Model file for the job. Use its own axes, mm. A direction names the side the tool comes from. Give positions to 0.01 mm unless a question says otherwise; leave off trailing zeros. Write each loop counter-clockwise with the first axis right and the second up, starting at its lowest first coordinate (ties: lowest second). Pieces come first, ordered by that corner, then holes. Notation, with made-up numbers: (63.25, -27) - (111.25, -27) arc R22 ccw to (111.25, -5) - close; hole circle Ø11 at (87.5, 3). An arc over 180 degrees is marked (long way). Use CSV: the item, a comma, the result in double quotes.
from build123d import *

# Parameters (mm, degrees)
EXTRUDE006_DEPTH                     = 2
EXTRUDE006_ONTO_SKETCH006_ROLL_ANGLE = 90
EXTRUDE006_PLACEMENT_ANGLE           = 90
SKETCH_W                             = 14.047477
SKETCH_H                             = 45.6
EXTRUDE004_DEPTH                     = 10
SKETCH002_R                          = 1.2
EXTRUDE001_DEPTH                     = 2
EXTRUDE005_DEPTH                     = 10
EXTRUDE003_DEPTH                     = 0.7
EXTRUDE003_DEPTH_BACK                = 0.2
FILLET_R                             = 0.2
CHAMFER_SIZE                         = 0.2
EXTRUDE002_DEPTH                     = 2
EXTRUDE_DEPTH                        = 1.6
EXTRUDE_DEPTH_BACK                   = 6.8


with BuildPart() as extrude006:
    # Sketch006 as drawn → Extrude006 (new, symmetric)
    with BuildSketch(Plane.XY):
        Polygon((-3.8, 0), (-2.9, 0.8), (2.9, 0.8), (3.8, 0), align=None)
    extrude(amount=EXTRUDE006_DEPTH, both=True)


with BuildPart() as extrude006_1:
    # Extrude006 onto Sketch006 roll: moved
    add(extrude006.part.rotate(Axis((0, 0, 0), (1, 0, 0)), EXTRUDE006_ONTO_SKETCH006_ROLL_ANGLE))


with BuildPart() as extrude006_2:
    # Extrude006 onto Sketch006 placement: moved
    add(extrude006_1.part)


with BuildPart() as extrude006_3:
    # Extrude006 placement: moved
    add(extrude006_2.part.moved(Location((50, 9.5, -6.8))).rotate(Axis((50, 9.5, -6.8), (0, 0, 1)), EXTRUDE006_PLACEMENT_ANGLE))


with BuildPart() as extrude004:
    # Sketch → Extrude004 (new body)
    with BuildSketch(Plane.XY):
        with Locations((51.252235, 25)):
            Rectangle(SKETCH_W, SKETCH_H)
    extrude(amount=EXTRUDE004_DEPTH)


with BuildPart() as extrude001:
    # Sketch002 → Extrude001 (new body)
    with BuildSketch(Plane.XY):
        with BuildLine():
            Line((4.8, 47), (4.8, 51))
            Line((4.8, 51), (9.2, 51))
            Line((9.2, 51), (9.2, 47.000001))
            ThreePointArc((4.8, 47), (7, 44.8), (9.2, 47.000001))
        make_face()
        with Locations((7, 47)):
            Circle(SKETCH002_R, mode=Mode.SUBTRACT)
        with BuildLine():
            ThreePointArc((9.2, 3), (7, 5.2), (4.8, 3))
            Line((4.8, 3), (4.8, -1))
            Line((4.8, -1), (9.2, -1))
            Line((9.2, -1), (9.2, 3))
        make_face()
        with Locations((7, 3)):
            Circle(SKETCH002_R, mode=Mode.SUBTRACT)
        with BuildLine():
            Line((40.8, 47), (40.8, 51))
            Line((40.8, 51), (45.2, 51))
            Line((45.2, 51), (45.2, 46.999987))
            ThreePointArc((40.8, 47), (42.999993, 44.8), (45.2, 46.999987))
        make_face()
        with Locations((43, 47)):
            Circle(SKETCH002_R, mode=Mode.SUBTRACT)
        with BuildLine():
            ThreePointArc((45.2, 3), (43, 5.2), (40.8, 3))
            Line((40.8, 3), (40.8, -1))
            Line((40.8, -1), (45.2, -1))
            Line((45.2, -1), (45.2, 3))
        make_face()
        with Locations((43, 3)):
            Circle(SKETCH002_R, mode=Mode.SUBTRACT)
    extrude(amount=-EXTRUDE001_DEPTH)


with BuildPart() as extrude005:
    # Sketch005 → Extrude005 (new body)
    with BuildSketch(Plane.XY):
        Polygon((8, 53), (8, 45), (-3, 45), (-3, 5), (8, 5), (8, -3), (42, -3), (42, 5), (53, 5), (53, 45), (42, 45), (42, 53), align=None)
    extrude(amount=EXTRUDE005_DEPTH)


with BuildPart() as cut003:
    # Sketch004 → Extrude003 (new body, two sides)
    with BuildSketch(Plane.XY) as extrude003_sk:
        with BuildLine():
            Line((2.3, 50.6), (47.7, 50.6))
            ThreePointArc((50.6, 47.7), (49.75061, 49.75061), (47.7, 50.6))
            Line((50.6, 47.7), (50.6, 2.3))
            ThreePointArc((47.7, -0.6), (49.75061, 0.24939), (50.6, 2.3))
            Line((47.7, -0.6), (2.3, -0.6))
            ThreePointArc((-0.6, 2.3), (0.24939, 0.24939), (2.3, -0.6))
            Line((-0.6, 2.3), (-0.6, 47.7))
            ThreePointArc((2.3, 50.6), (0.24939, 49.75061), (-0.6, 47.7))
        make_face()
        with BuildLine():
            Line((2.3, 50), (47.7, 50))
            ThreePointArc((50, 47.7), (49.326346, 49.326346), (47.7, 50))
            Line((50, 47.7), (50, 2.3))
            ThreePointArc((47.7, 0), (49.326346, 0.673654), (50, 2.3))
            Line((47.7, 0), (2.3, 0))
            ThreePointArc((0, 2.3), (0.673654, 0.673654), (2.3, 0))
            Line((0, 2.3), (0, 47.7))
            ThreePointArc((2.3, 50), (0.673654, 49.326346), (0, 47.7))
        make_face(mode=Mode.SUBTRACT)
    extrude(amount=EXTRUDE003_DEPTH)
    extrude(extrude003_sk.sketch, amount=-EXTRUDE003_DEPTH_BACK)


with BuildPart() as cut003_1:
    # Extrude003 placement: moved
    add(cut003.part.moved(Location((0, 0, 1.6))))

    # Fillet
    fillet_edges = [cut003_1.edges().sort_by_distance(p)[0] for p in [
        (-0.6, 25, 2.3),
        (0.24939, 49.75061, 2.3),
        (25, 50.6, 2.3),
        (49.75061, 49.75061, 2.3),
        (50.6, 25, 2.3),
        (49.75061, 0.24939, 2.3),
        (25, -0.6, 2.3),
        (0.24939, 0.24939, 2.3),
    ]]
    fillet(fillet_edges, radius=FILLET_R)

    # Chamfer
    chamfer_edges = [cut003_1.edges().sort_by_distance(p)[0] for p in [
        (0, 25, 1.4),
        (0.673654, 49.326346, 1.4),
        (25, 50, 1.4),
        (49.326346, 49.326346, 1.4),
        (50, 25, 1.4),
        (49.326346, 0.673654, 1.4),
        (25, 0, 1.4),
        (0.673654, 0.673654, 1.4),
    ]]
    chamfer(chamfer_edges, length=CHAMFER_SIZE)

    # Cut003: cut Extrude005
    add(extrude005.part, mode=Mode.SUBTRACT)


with BuildPart() as extrude002:
    # Sketch003 → Extrude002 (new body)
    with BuildSketch(Plane.XY):
        with BuildLine():
            Line((2.3, 51.1), (9, 51.1))
            Line((9, 44), (9, 51.1))
            Line((-1.1, 44), (9, 44))
            Line((-1.1, 44), (-1.1, 47.654452))
            ThreePointArc((2.3, 51.1), (-0.12032, 50.088024), (-1.1, 47.654452))
        make_face()
        with BuildLine():
            Line((51.1, 47.699699), (51.1, 44))
            Line((41, 44), (51.1, 44))
            Line((41, 51.1), (41, 44))
            Line((41, 51.1), (47.698586, 51.1))
            ThreePointArc((51.1, 47.699699), (50.103681, 50.104468), (47.698586, 51.1))
        make_face()
        with BuildLine():
            Line((47.6997, -1.1), (41, -1.1))
            Line((41, -1.1), (41, 6))
            Line((41, 6), (51.1, 6))
            Line((51.1, 6), (51.1, 2.297304))
            ThreePointArc((47.6997, -1.1), (50.103016, -0.105134), (51.1, 2.297304))
        make_face()
        with BuildLine():
            Line((-1.1, 2.300296), (-1.1, 6))
            Line((-1.1, 6), (9, 6))
            Line((9, 6), (9, -1.1))
            Line((9, -1.1), (2.294563, -1.1))
            ThreePointArc((-1.1, 2.300296), (-0.106103, -0.10205), (2.294563, -1.1))
        make_face()
    extrude(amount=-EXTRUDE002_DEPTH)


with BuildPart() as extrude002_1:
    # Extrude002 placement: moved
    add(extrude002.part.moved(Location((0, 0, -5.6))))


with BuildPart() as cut004:
    # Sketch001 → Extrude (new body, two sides)
    with BuildSketch(Plane.XY) as extrude_sk:
        with BuildLine():
            Line((2.3, 52), (47.7, 52))
            ThreePointArc((52, 47.7), (50.740559, 50.740559), (47.7, 52))
            Line((52, 47.7), (52, 2.3))
            ThreePointArc((47.7, -2), (50.740559, -0.740559), (52, 2.3))
            Line((47.7, -2), (2.3, -2))
            ThreePointArc((-2, 2.3), (-0.740559, -0.740559), (2.3, -2))
            Line((-2, 2.3), (-2, 47.7))
            ThreePointArc((2.3, 52), (-0.740559, 50.740559), (-2, 47.7))
        make_face()
        with BuildLine():
            Line((2.3, 50.1), (47.7, 50.1))
            ThreePointArc((50.1, 47.7), (49.397056, 49.397056), (47.7, 50.1))
            Line((50.1, 47.7), (50.1, 2.3))
            ThreePointArc((47.7, -0.1), (49.397056, 0.602944), (50.1, 2.3))
            Line((47.7, -0.1), (2.3, -0.1))
            ThreePointArc((-0.1, 2.3), (0.602944, 0.602944), (2.3, -0.1))
            Line((-0.1, 2.3), (-0.1, 47.7))
            ThreePointArc((2.3, 50.1), (0.602944, 49.397056), (-0.1, 47.7))
        make_face(mode=Mode.SUBTRACT)
    extrude(amount=EXTRUDE_DEPTH)
    extrude(extrude_sk.sketch, amount=-EXTRUDE_DEPTH_BACK)

    # Cut002: cut Extrude002
    add(extrude002_1.part, mode=Mode.SUBTRACT)

    # Fusion001: union Cut003
    add(cut003_1.part)

    # Fusion002: union Extrude001
    add(extrude001.part)

    # Cut: cut Extrude004
    add(extrude004.part, mode=Mode.SUBTRACT)

    # Cut004: cut Extrude006
    add(extrude006_3.part, mode=Mode.SUBTRACT)


solid = cut004.part
(1) 3-axis set-ups, long thin cutter, end or side, ignore diameter. For faces 1 (the face through (50.71, -0.77, -2.54)), 2 (the face through (50.1, 25, -3)), 3 (the face through (49, 50, -5.6)): which of +Z, -Z, +X, -X, +Y, -Y reach the whole face in a straight line?
Checked values:
face 1,"+Z, -Z, +X, -Y"
face 2,"+Z, -Z"
face 3,"-Z"
(2) Saw through at D-D, the plane x = 38.5. List the corners of the cut face in (y, z).
Checked values:
outline,"(-2, -6.8) - (-0.1, -6.8) - (-0.1, 1.6) - (-2, 1.6) - close; (50.1, -6.8) - (52, -6.8) - (52, 1.6) - (50.1, 1.6) - close"
(3) Saw through at A-A, the plane y = 9.5. List the corners of the cut face in (x, z), then the cut area to 3 significant figures.
Checked values:
outline,"(-2, -6.8) - (-0.1, -6.8) - (-0.1, 1.6) - (-2, 1.6) - close; (50.1, -6) - (52, -6) - (52, 0) - (50.1, 0) - close"
area,"27.4 mm^2"
(4) Saw through at B-B, the plane x = 46. List the corners of the cut face in (y, z), then the cut area to 3 significant figures.
Checked values:
outline,"(-2, -6.8) - (-1.1, -6.8) - (-1.1, -5.6) - (-0.1, -5.6) - (-0.1, 1.5) - (0, 1.6) - (0, 2.3) - (-0.4, 2.3) arc R0.2 ccw to (-0.6, 2.1) - (-0.6, 1.6) - (-2, 1.6) - close; (50, 1.6) - (50.1, 1.5) - (50.1, -5.6) - (51.1, -5.6) - (51.1, -6.8) - (52, -6.8) - (52, 1.6) - (50.6, 1.6) - (50.6, 2.1) arc R0.2 ccw to (50.4, 2.3) - (50, 2.3) - close"
area,"30.4 mm^2"
(5) Flat gauge pins, fed straight in: P1, Ø0.6, axis at x = 51.5, z = 1.5, coming from the -Y side; P2, Ø2, axis at x = 7.5, y = 4, coming from the -Z side; P3, Ø0.5, axis at y = -0.5, z = 2, coming from the +X side; P4, Ø1.9, axis at x = 7, y = 3, coming from the -Z side. Where does each tip first touch, or does it go through?
Checked values:
P1,"stops at y = -0.2"
P2,"stops at z = -2"
P3,"stops at x = 49.08"
P4,"passes through"
(6) Pull direction X, two halves, no side cores. Call faces 4 (the face through (-1.1, 4, -6)), 5 (the face through (49.7, 0.2, 1.9)), 6 (the face through (51, 9, -6)): released by +X, released by -X, zero draft, split by the parting line, or undercut.
Checked values:
face 4,"undercut"
face 5,"released by +X"
face 6,"zero draft"
(7) Saw through at C-C, the plane z = -4.75. List the corners of the cut face in (x, y).
Checked values:
outline,"(-2, 2.3) arc R4.3 ccw to (2.3, -2) - (47.7, -2) arc R4.3 ccw to (52, 2.3) - (52, 47.7) arc R4.3 ccw to (47.7, 52) - (2.3, 52) arc R4.3 ccw to (-2, 47.7) - close; hole (-0.1, 2.3) arc R2.4 ccw to (2.3, -0.1) - (47.7, -0.1) arc R2.4 ccw to (50.1, 2.3) - (50.1, 47.7) arc R2.4 ccw to (47.7, 50.1) - (2.3, 50.1) arc R2.4 ccw to (-0.1, 47.7) - close"
(8) Wall check: probe 1 along Y at (x, z) = (43, -1.1); probe 2 along X at (y, z) = (12.5, -1.75). Give the ranges that are in metal, low to high. Write a range as [from, to].
Checked values:
probe 1,"y = [-2, 1.8], [4.2, 5.2], [44.8, 45.8], [48.2, 52]"
probe 2,"x = [-2, -0.1], [50.1, 52]"
